Autodesk Inventor part; units mm, degrees
ref_plane "YZ Plane" through (0, 0, 0) normal (1, 0, 0) x (0, 1, 0)
ref_plane "XZ Plane" through (0, 0, 0) normal (0, 1, 0) x (-1, 0, 0)
ref_plane "XY Plane" through (0, 0, 0) normal (0, 0, 1) x (1, 0, 0)
sketch "Sketch1" plane through (0, 0, 0) normal (1, 0, 0) x (0, 1, 0)
  circle A0 centre (0, 0) radius 5.0038
  circle A1 centre (0, 0) radius 4.0005
  dimension "d0" = 10.0076
  dimension "d1" = 8.001
extrude "Extrusion1" add sketch "Sketch1" along normal blind 11.5062
sketch "Sketch2" plane through (11.5062, 0, 0) normal (1, 0, 0) x (0, 0, -1)
  circle A0 centre (0, 0) radius 12.7
  circle A1 centre (0, 0) radius 4.0005
  dimension "d4" = 25.4
  dimension "d7" = 8.001
extrude "Extrusion2" add sketch "Sketch2" along normal blind 12.7
chamfer "Chamfer2" distance 0.254 angle 45 1 edges at (0, -4.0005, 0)
properties part number "DTR-2"
Read the model definition and answer for the solid it produces. Units are mm, in the model's axes. A direction names the side the tool comes from. Give positions to 0.01 mm unless a question says otherwise; leave off trailing zeros. Write each loop counter-clockwise with the first axis right and the second up, starting at its lowest first coordinate (ties: lowest second). Pieces come first, ordered by that corner, then holes. Notation, with made-up numbers: (85, 14.25) - (143, 14.25) arc R18 ccw to (143, 20.25) - close; hole circle Ø8 at (-37, -38). An arc over 180 degrees is marked (long way). Answer in a Markdown table with one row per item. Add a question column.
Item 1: Section A-A, the plane y = 0 is taken. Write down the section's boundary in (x, z).
Item 2: Section C-C, the plane x = 12 is taken. Write down the section's boundary in (y, z).
Item 3: Flat-ended cylindrical pins translate along their axes: P1, Ø8, axis at x = 19, z = 8.5, coming from the -Y side; P2, Ø1.5, axis at x = 4, z = -1, coming from the -Y side; P3, Ø8, axis at x = 11, z = -7.5, coming from the +Y side. Find the tip coordinate at first contact, or state that the pin passes through.
Item 4: A tool of negligible diameter and unlimited length cuts with its end or side. For faces 1 (the face through (5.673, -3.971, 3.045)), 2 (the face through (24.206, 3, 3)), from which of +Z, -Z, +X, -X, +Y, -Y can it reach the whole face along a straight path? Write none if from no direction.
Item 5: Determine the mould class of faces 3 (the face through (12.06, -2.11, -3.4)), 4 (the face through (11.506, 0.2, -5.5)), 5 (the face through (17.77, 12.4, 2.75)) for opening direction Y: pulls with the +Y half, pulls with the -Y half, needs draft (parallel to the pull), parting line crosses it, or undercut.
Item 6: Section D-D, the plane y = 10.5 is taken. Write down the section's boundary in (x, z), and give its area (3 significant figures).
Item 7: Find the intervals of material crossed by L1, parallel to Y at x = 16.75, z = 0; L2, parallel to Y at x = 7.25, z = 0.25; L3, parallel to Z at x = 8.75, y = 0, in increasing order.
Recorded:
| question | item | result |
|---|---|---|
| 1 | outline | (0, -5) - (11.51, -5) - (11.51, -12.7) - (24.21, -12.7) - (24.21, -4) - (0.25, -4) - (0, -4.25) - close; (0, 4.25) - (0.25, 4) - (24.21, 4) - (24.21, 12.7) - (11.51, 12.7) - (11.51, 5) - (0, 5) - close |
| 2 | outline | circle Ø25.4 at (0, 0); hole circle Ø8 at (0, 0) |
| 3 | P1 | stops at y = -11.88 |
| 3 | P2 | stops at y = -5 |
| 3 | P3 | stops at y = 12.2 |
| 4 | face 1 | -X |
| 4 | face 2 | +Z, -Z, +X, +Y, -Y |
| 5 | face 3 | undercut |
| 5 | face 4 | needs draft |
| 5 | face 5 | parting line crosses it |
| 6 | outline | (11.51, -7.14) - (24.21, -7.14) - (24.21, 7.14) - (11.51, 7.14) - close |
| 6 | area | 181 mm2 |
| 7 | L1 | y = -12.7 to -4, 4 to 12.7 |
| 7 | L2 | y = -5 to -3.99, 3.99 to 5 |
| 7 | L3 | z = -5 to -4, 4 to 5 |
